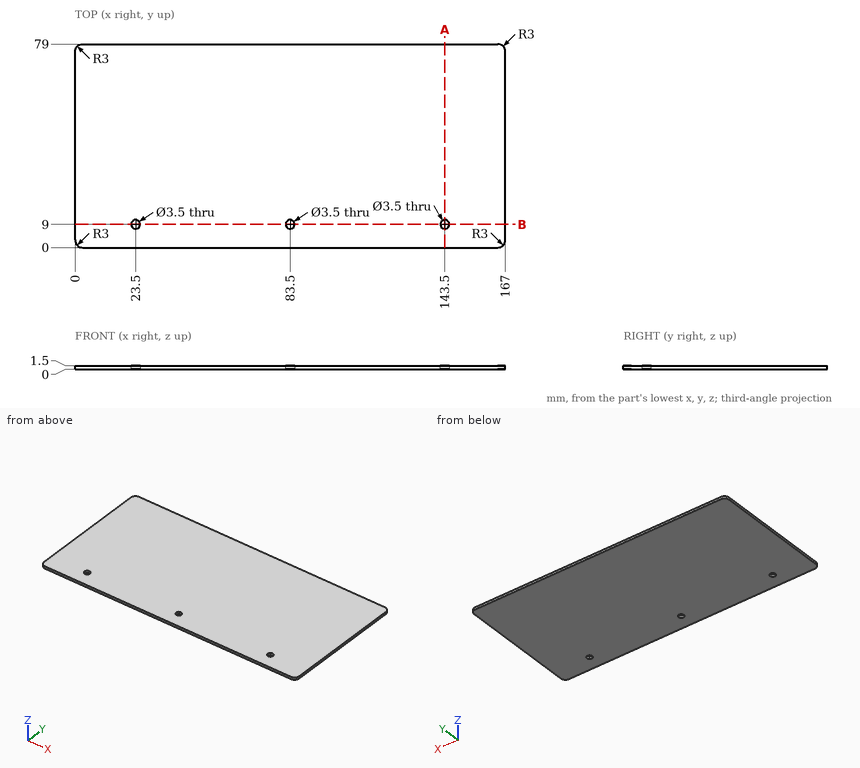
Geometry check sheet. Reference: drawing and pictorial views, mm from the part's lowest x, y, z. Round coordinates to 2 decimals unless told otherwise and drop trailing zeros. Order: outer loops, then holes, each group sorted by start corner. A loop starts at its lowest first (then second) coordinate and runs counter-clockwise, first axis right, second up. Notation, with made-up numbers: (-6, 16) -> (38, 16) arc R15 cw to (38, 33) -> close; hole circle Ø6 at (1, 40). An arc over 180 degrees is marked (long way). One line per item, written item: value. Start each with the question number.
Q1. Cross-section at A-A (x = 143.5). Record the boundary of the cut face in (y, z).
Q2. Gauge pin test, flat end, axial feed: pin 1 Ø3 at (x, y) = (143.5, 9) entering from +Z. Record the tip position at first contact, or that the pin passes through.
Q3. Thickness scan on line 1 (Y direction, x = 83.5, z = 0.5). Record the ranges inside material, lowest first.
Q4. Cross-section at B-B (y = 9). Record the boundary of the cut face in (x, z), and give its area (3 significant figures).
Completed:
1. outline: (0, 0) -> (7.25, 0) -> (7.25, 1.5) -> (0, 1.5) -> close; (10.75, 0) -> (79, 0) -> (79, 1.5) -> (10.75, 1.5) -> close
2. pin 1: passes through
3. line 1: y = 0 to 7.25, 10.75 to 79
4. outline: (0, 0) -> (21.75, 0) -> (21.75, 1.5) -> (0, 1.5) -> close; (25.25, 0) -> (81.75, 0) -> (81.75, 1.5) -> (25.25, 1.5) -> close; (85.25, 0) -> (141.75, 0) -> (141.75, 1.5) -> (85.25, 1.5) -> close; (145.25, 0) -> (167, 0) -> (167, 1.5) -> (145.25, 1.5) -> close
4. area: 235 mm²
